Input: dimensioned drawing with shaded views. Units: mm. Origin: part minimum x, y, z. A direction names the side the tool comes from. Give positions to 0.01 mm unless a question says otherwise; leave off trailing zeros. Loops run counter-clockwise (first coordinate to the right, second up) from the corner with the lowest first, then second, coordinate; pieces in that order, holes last. Notation, with made-up numbers: (-36, -36) -> (-32, -36) arc R16 cw to (-32, -10) -> close; hole circle Ø4 at (0, -15.5). An arc over 180 degrees is marked (long way). Answer in a Markdown table with one row per item. Add a question column.
1) First-contact query: P1, Ø8.5, axis at x = 9.81, y = 9.81, coming from the +Z side; P2, Ø4, axis at x = 12, y = 10, coming from the -Z side; P3, Ø2, axis at x = 15.06, y = 9.81, coming from the -Z side. Flat tips, straight axial feed; report the tip coordinate or a pass-through.
2) Line query: line 1 (X direction, y = 9.25, z = 1.9) (1 decimal); line 2 (Y direction, x = 9.75, z = 4.7); line 3 (Y direction, x = 11.75, z = 4.4) (1 decimal). Output: solid intervals per line, ascending. Write a range as from..to.
3) Draft query along X for the marked faces 4, 5 and 6. Return one class per face: +X half, -X half, draft (parallel to the pull), parting line (faces both ways), or undercut.
4) Section query B-B (x = 10). Return the cut outline in (y, z).
5) Section query D-D (y = 9.25). Give the number of separate pieces and of enclosed holes in the cut face.
6) Access query for the marked faces 1, 2 and 3. Directions: +Z, -Z, +X, -X, +Y, -Y. A direction counts if a zero-diameter tool reaches every point of the face in a straight line with its end or side. Return the directions, or none.
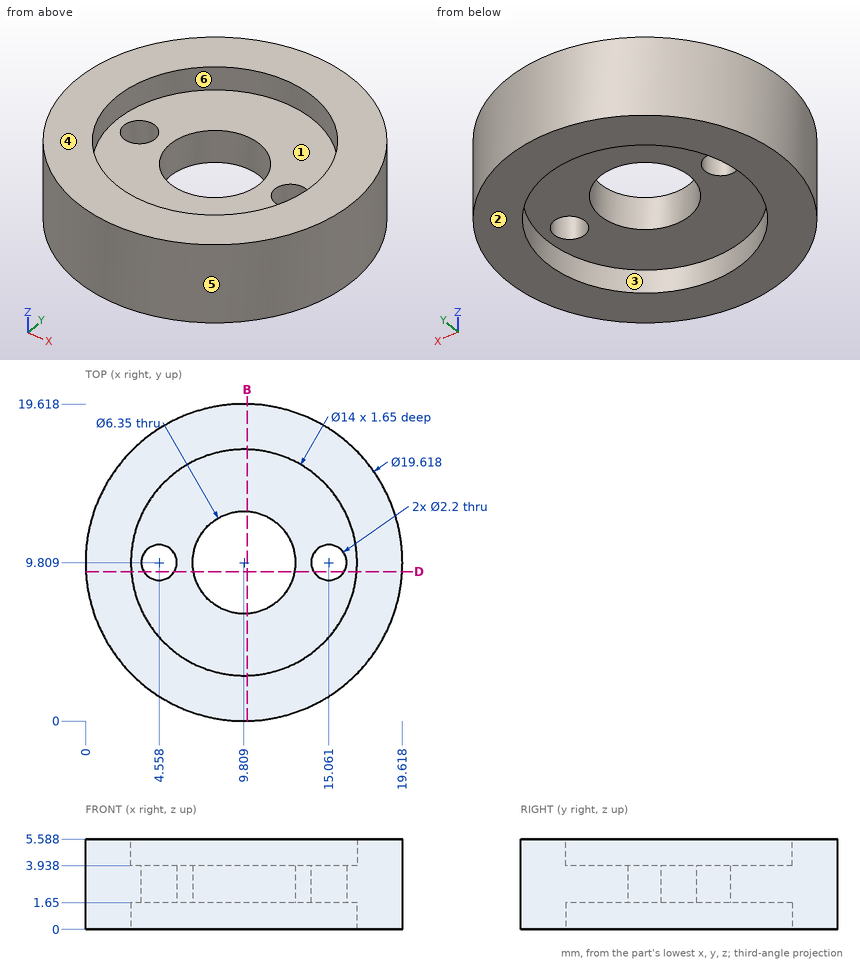
Evaluation:
| question | item | result |
|---|---|---|
| 1 | P1 | z = 3.94 |
| 1 | P2 | z = 1.65 |
| 1 | P3 | through |
| 2 | line 1 | 0..3.6, 5.5..6.7, 12.9..14.1, 16..19.6 |
| 2 | line 2 | 0..2.81, 16.81..19.62 |
| 2 | line 3 | 0.2..3.1, 16.5..19.4 |
| 3 | face 4 | draft |
| 3 | face 5 | parting line |
| 3 | face 6 | undercut |
| 4 | outline | (0, 0) -> (2.81, 0) -> (2.81, 1.65) -> (6.64, 1.65) -> (6.64, 3.94) -> (2.81, 3.94) -> (2.81, 5.59) -> (0, 5.59) -> close; (12.98, 1.65) -> (16.81, 1.65) -> (16.81, 0) -> (19.62, 0) -> (19.62, 5.59) -> (16.81, 5.59) -> (16.81, 3.94) -> (12.98, 3.94) -> close |
| 5 | separate pieces | 4 |
| 5 | enclosed holes | 0 |
| 6 | face 1 | +Z |
| 6 | face 2 | -Z, +X, -X, +Y, -Y |
| 6 | face 3 | -Z |
